Design review of the part built by this model. Coordinates are the model's own, in mm. Face numbers are marked on the shaded views. A direction names the side the tool comes from. Round coordinates to 2 decimals unless told otherwise and drop trailing zeros. Write each loop counter-clockwise with the first axis right and the second up, starting at its lowest first coordinate (ties: lowest second). Pieces come first, ordered by that corner, then holes. Notation, with made-up numbers: (35, -28.75) - (75, -28.75) arc R25 ccw to (75, 0.25) - close; hole circle Ø10 at (-1.75, -18). An arc over 180 degrees is marked (long way). Use one line per item in the form item = value.
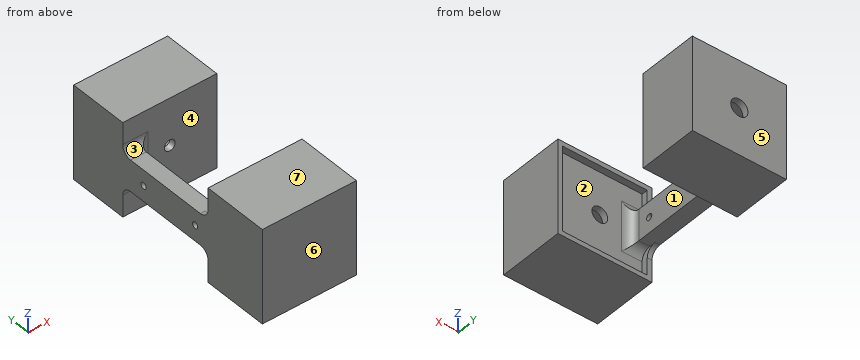
```python
from build123d import *

# Parameters (mm, degrees)
SKETCH_2_W          = 30
SKETCH_2_H          = 30
EXTRUDE_1_DEPTH     = 2
SKETCH_3_W          = 30
SKETCH_3_H          = 30
SKETCH_3_W_2        = 26
SKETCH_3_H_2        = 26
EXTRUDE_2_DEPTH     = 15
SKETCH_4_W          = 30
SKETCH_4_H          = 30
SKETCH_4_W_2        = 27
SKETCH_4_H_2        = 27
EXTRUDE_3_DEPTH     = 2
SKETCH_5_W          = 5
SKETCH_5_H          = 10
EXTRUDE_2_2_DEPTH   = 35
SKETCH_6_R          = 1
CUT_EXTRUDE_1_DEPTH = 50.939963957
SKETCH_8_R          = 2.5
CUT_EXTRUDE_2_DEPTH = 41.926763859
FILLET_1_R          = 3
FILLET_2_R          = 3
SKETCH_9_W          = 30
SKETCH_9_H          = 30
EXTRUDE_3_2_DEPTH   = 2
SKETCH_10_W         = 30
SKETCH_10_H         = 30
SKETCH_10_W_2       = 26
SKETCH_10_H_2       = 26
EXTRUDE_4_DEPTH     = 15
SKETCH_11_R         = 1.75
CUT_EXTRUDE_3_DEPTH = 3
FILLET_3_R          = 3
SKETCH_13_W         = 30
SKETCH_13_H         = 30
EXTRUDE_4_2_DEPTH   = 2
SKETCH_14_W         = 30
SKETCH_14_H         = 30
EXTRUDE_5_DEPTH     = 2
SKETCH_15_R         = 2.75
CUT_EXTRUDE_4_DEPTH = 2


with BuildPart() as part:
    # Эскиз2 → Бобышка-Вытянуть1 (new body)
    with BuildSketch(Plane(origin=(0, 0, 0), x_dir=(1, 0, 0), z_dir=(0, 1, 0))):
        Rectangle(SKETCH_2_W, SKETCH_2_H)
    extrude(amount=EXTRUDE_1_DEPTH)

    # Эскиз3 → Extrude 2 (add)
    with BuildSketch(Plane.XZ):
        Rectangle(SKETCH_3_W, SKETCH_3_H)
        Rectangle(SKETCH_3_W_2, SKETCH_3_H_2, mode=Mode.SUBTRACT)
    extrude(amount=EXTRUDE_2_DEPTH)

    # Эскиз4 → Extrude 3 (add)
    with BuildSketch(Plane(origin=(0, 2, 0), x_dir=(1, 0, 0), z_dir=(0, 1, 0))):
        Rectangle(SKETCH_4_W, SKETCH_4_H)
        Rectangle(SKETCH_4_W_2, SKETCH_4_H_2, mode=Mode.SUBTRACT)
    extrude(amount=EXTRUDE_3_DEPTH)

    # Эскиз5 → Extrude 2 2 (add)
    with BuildSketch(Plane(origin=(0, 2, 0), x_dir=(1, 0, 0), z_dir=(0, 1, 0))):
        with Locations((-12.5, 0)):
            Rectangle(SKETCH_5_W, SKETCH_5_H)
    extrude(amount=EXTRUDE_2_2_DEPTH)

    # Эскиз6 → Вырез-Вытянуть1 (cut, through all)
    with BuildSketch(Plane.ZY.offset(15)):
        with Locations((0, 29)):
            Circle(SKETCH_6_R)
        with Locations((0, 9)):
            Circle(SKETCH_6_R)
    extrude(amount=-CUT_EXTRUDE_1_DEPTH, mode=Mode.SUBTRACT)

    # Эскиз8 → Вырез-Вытянуть2 (cut, through all)
    with BuildSketch(Plane(origin=(0, 2, 0), x_dir=(1, 0, 0), z_dir=(0, 1, 0))):
        with Locations(Location((0, 0, 0), (0, 0, 270))):
            Circle(SKETCH_8_R)
    extrude(amount=-CUT_EXTRUDE_2_DEPTH, mode=Mode.SUBTRACT)

    # Скругление1
    # the kernel refuses this fillet: 3 mm, written as the material it adds along each edge
    with BuildSketch(Plane(origin=(-10, 2, -5), x_dir=(1, 0, 0), z_dir=(0, 0, 1))) as fillet_1_piece_1:
        with BuildLine():
            CenterArc((FILLET_1_R, FILLET_1_R), FILLET_1_R, 180, 90)
            Line((0, FILLET_1_R), (0, 0))
            Line((0, 0), (FILLET_1_R, 0))
        make_face()
    extrude(amount=10)
    with BuildSketch(Plane(origin=(-21, 2, -5), x_dir=(0, 1, 0), z_dir=(1, 0, 0))) as fillet_1_piece_2_section:
        with BuildLine():
            CenterArc((FILLET_1_R, -FILLET_1_R), FILLET_1_R, 90, 90)
            Line((0, -FILLET_1_R), (0, 0))
            Line((0, 0), (FILLET_1_R, 0))
        make_face()
    fillet_1_piece_2 = extrude(amount=11, mode=Mode.PRIVATE)
    fillet_1_piece_2 = split(fillet_1_piece_2, bisect_by=Plane(origin=(-15, 2, -5), z_dir=(1, 0, 0)), keep=Keep.TOP, mode=Mode.PRIVATE)
    add(fillet_1_piece_2)
    with BuildSketch(Plane(origin=(-10, 2, 5), x_dir=(0, 1, 0), z_dir=(-1, 0, 0))) as fillet_1_piece_3_section:
        with BuildLine():
            CenterArc((FILLET_1_R, -FILLET_1_R), FILLET_1_R, 90, 90)
            Line((0, -FILLET_1_R), (0, 0))
            Line((0, 0), (FILLET_1_R, 0))
        make_face()
    fillet_1_piece_3 = extrude(amount=11, mode=Mode.PRIVATE)
    fillet_1_piece_3 = split(fillet_1_piece_3, bisect_by=Plane(origin=(-15, 2, 5), z_dir=(1, 0, 0)), keep=Keep.TOP, mode=Mode.PRIVATE)
    add(fillet_1_piece_3)
    with BuildSketch(Plane(origin=(-13.5, 2, -5), x_dir=(0, 1, 0), z_dir=(1, 0, 0))) as fillet_1_piece_4a_section:
        with BuildLine():
            CenterArc((FILLET_1_R, -FILLET_1_R), FILLET_1_R, 90, 90)
            Line((0, -FILLET_1_R), (0, 0))
            Line((0, 0), (FILLET_1_R, 0))
        make_face()
    fillet_1_piece_4a = extrude(amount=11, mode=Mode.PRIVATE)
    fillet_1_piece_4a = split(fillet_1_piece_4a, bisect_by=Plane(origin=(-10, 2, -5), z_dir=(1, 0, 0)), keep=Keep.TOP, mode=Mode.PRIVATE)
    with BuildSketch(Plane(origin=(-10, 2, -12.5), x_dir=(1, 0, 0), z_dir=(0, 0, 1))) as fillet_1_piece_4b_section:
        with BuildLine():
            CenterArc((FILLET_1_R, FILLET_1_R), FILLET_1_R, 180, 90)
            Line((0, FILLET_1_R), (0, 0))
            Line((0, 0), (FILLET_1_R, 0))
        make_face()
    fillet_1_piece_4b = extrude(amount=17.5, mode=Mode.PRIVATE)
    fillet_1_piece_4b = split(fillet_1_piece_4b, bisect_by=Plane(origin=(-10, 2, -5), z_dir=(0, 0, -1)), keep=Keep.TOP, mode=Mode.PRIVATE)
    fillet_1_piece_4 = fillet_1_piece_4a & fillet_1_piece_4b
    add(fillet_1_piece_4)
    with BuildSketch(Plane(origin=(-2.5, 2, 5), x_dir=(0, 1, 0), z_dir=(-1, 0, 0))) as fillet_1_piece_5a_section:
        with BuildLine():
            CenterArc((FILLET_1_R, -FILLET_1_R), FILLET_1_R, 90, 90)
            Line((0, -FILLET_1_R), (0, 0))
            Line((0, 0), (FILLET_1_R, 0))
        make_face()
    fillet_1_piece_5a = extrude(amount=11, mode=Mode.PRIVATE)
    fillet_1_piece_5a = split(fillet_1_piece_5a, bisect_by=Plane(origin=(-10, 2, 5), z_dir=(1, 0, 0)), keep=Keep.TOP, mode=Mode.PRIVATE)
    with BuildSketch(Plane(origin=(-10, 2, -5), x_dir=(1, 0, 0), z_dir=(0, 0, 1))) as fillet_1_piece_5b_section:
        with BuildLine():
            CenterArc((FILLET_1_R, FILLET_1_R), FILLET_1_R, 180, 90)
            Line((0, FILLET_1_R), (0, 0))
            Line((0, 0), (FILLET_1_R, 0))
        make_face()
    fillet_1_piece_5b = extrude(amount=17.5, mode=Mode.PRIVATE)
    fillet_1_piece_5b = split(fillet_1_piece_5b, bisect_by=Plane(origin=(-10, 2, 5), z_dir=(0, 0, 1)), keep=Keep.TOP, mode=Mode.PRIVATE)
    fillet_1_piece_5 = fillet_1_piece_5a & fillet_1_piece_5b
    add(fillet_1_piece_5)

    # Скругление2
    # the kernel refuses this fillet: 3 mm, written as the material it adds along each edge
    with BuildSketch(Plane(origin=(-13.5, 4, -5.171572875), x_dir=(0, 0.9983685980477195, 0.0570976569767209), z_dir=(-1, 0, 0)), Plane(origin=(-15, 4, 5.171572875), x_dir=(0, 0.9983685980477195, -0.0570976569767209), z_dir=(1, 0, 0))) as fillet_2_piece_1:
        with BuildLine():
            CenterArc((2.833609232, 2.995105794), FILLET_2_R, 183.273234946, 90)
            Line((-0.161496562, 2.823812823), (-0.461007141, 2.806683526))
            Line((-0.461007141, 2.806683526), (-0.299510579, -0.017129297))
            Line((-0.299510579, -0.017129297), (-0.083687204, -0.288091048))
            ThreePointArc((-0.083687204, -0.288091048), (1.025294304, -0.413705893), (3.0220315, -0.299510579))
            Line((3.0220315, -0.299510579), (3.004902203, 0))
        make_face()
    extrude(amount=1.5)

    # Эскиз9 → Extrude 3 2 (add)
    with BuildSketch(Plane(origin=(0, 37, 0), x_dir=(1, 0, 0), z_dir=(0, 1, 0))):
        Rectangle(SKETCH_9_W, SKETCH_9_H)
    extrude(amount=EXTRUDE_3_2_DEPTH)

    # Эскиз10 → Extrude 4 (add)
    with BuildSketch(Plane(origin=(0, 39, 0), x_dir=(1, 0, 0), z_dir=(0, 1, 0))):
        Rectangle(SKETCH_10_W, SKETCH_10_H)
        Rectangle(SKETCH_10_W_2, SKETCH_10_H_2, mode=Mode.SUBTRACT)
    extrude(amount=EXTRUDE_4_DEPTH)

    # Эскиз11 → Вырез-Вытянуть3 (cut)
    with BuildSketch(Plane(origin=(0, 39, 0), x_dir=(1, 0, 0), z_dir=(0, 1, 0))):
        with Locations(Location((0, 0, 0), (0, 0, 270))):
            Circle(SKETCH_11_R)
    extrude(amount=-CUT_EXTRUDE_3_DEPTH, mode=Mode.SUBTRACT)

    # Скругление3
    fillet_3_edges = [part.edges().sort_by_distance(p)[0] for p in [
        (-10, 37, 0),
        (-12.5, 37, -5),
        (-12.5, 37, 5),
    ]]
    fillet(fillet_3_edges, radius=FILLET_3_R)

    # Эскиз13 → Extrude 4 2 (add)
    with BuildSketch(Plane.XZ.offset(15)):
        Rectangle(SKETCH_13_W, SKETCH_13_H)
    extrude(amount=EXTRUDE_4_2_DEPTH)

    # Эскиз14 → Бобышка-Вытянуть5 (add)
    with BuildSketch(Plane(origin=(0, 54, 0), x_dir=(1, 0, 0), z_dir=(0, 1, 0))):
        Rectangle(SKETCH_14_W, SKETCH_14_H)
    extrude(amount=EXTRUDE_5_DEPTH)

    # Эскиз15 → Вырез-Вытянуть4 (cut)
    with BuildSketch(Plane(origin=(0, 56, 0), x_dir=(1, 0, 0), z_dir=(0, 1, 0))):
        with Locations(Location((0, 0, 0), (0, 0, 270))):
            Circle(SKETCH_15_R)
    extrude(amount=-CUT_EXTRUDE_4_DEPTH, mode=Mode.SUBTRACT)


solid = part.part
```
Q1. We need section B-B on x = 0. State how many separate pieces and enclosed holes the cut face has, then the cut area to 3 significant figures.
Calculated:
separate_pieces = 3
enclosed_holes = 0
area = 338 mm2
Q2. Draft analysis for pull direction Y (two halves, no side actions). For the marked faces 4, 5, 6 and 7, state which applies: released by +Y, released by -Y, zero draft, split by the parting line, or undercut.
Calculated:
face_4 = undercut
face_5 = released by +Y
face_6 = released by -Y
face_7 = zero draft
Q3. We need section A-A on z = 9.5. Write out the cut boundary in (x, y), then the cut area to 3 significant figures.
Calculated:
outline = (-15, -17) - (15, -17) - (15, 4) - (13.5, 4) - (13.5, 2) - (-13.5, 2) - (-13.5, 4) - (-15, 4) - close; (-15, 37) - (15, 37) - (15, 56) - (-15, 56) - close; hole (-13, -15) - (13, -15) - (13, 0) - (-13, 0) - close; hole (-13, 39) - (13, 39) - (13, 54) - (-13, 54) - close
area = 366 mm2
Q4. To check wall thickness, follow line 1 along Y through (x, z) = (-12.35, 0); line 2 along Y through (x, z) = (4.75, -0.5); line 3 along X through (y, z) = (47.5, 8.25). State the ranges of each line that lie inside material, in increasing order. Write a range as from..to.
Calculated:
line_1 = -17..-15, 0..8, 10..28, 30..39, 54..56
line_2 = -17..-15, 0..2, 37..39, 54..56
line_3 = -15..-13, 13..15
Q5. Machinability: for the marked faces 1, 2 and 3, which of the approach directions +Z, -Z, +X, -X, +Y, -Y give a long, thin tool a straight path to every point of the face, cutting with its end or side? Answer none if there is none.
Calculated:
face_1 = +Z, -Z, +X
face_2 = none
face_3 = +Z, +X, -X
Q6. We need section D-D on x = 7. Write out the cut boundary in (y, z).
Calculated:
outline = (-17, -15) - (4, -15) - (4, -13.5) - (2, -13.5) - (2, 13.5) - (4, 13.5) - (4, 15) - (-17, 15) - close; (37, -15) - (56, -15) - (56, 15) - (37, 15) - close; hole (-15, -13) - (0, -13) - (0, 13) - (-15, 13) - close; hole (39, -13) - (54, -13) - (54, 13) - (39, 13) - close
Q7. We need section C-C on y = 9. Write out the cut boundary in (x, z).
Calculated:
outline = (-15, -5) - (-10, -5) - (-10, -1) - (-15, -1) - close; (-15, 1) - (-10, 1) - (-10, 5) - (-15, 5) - close
